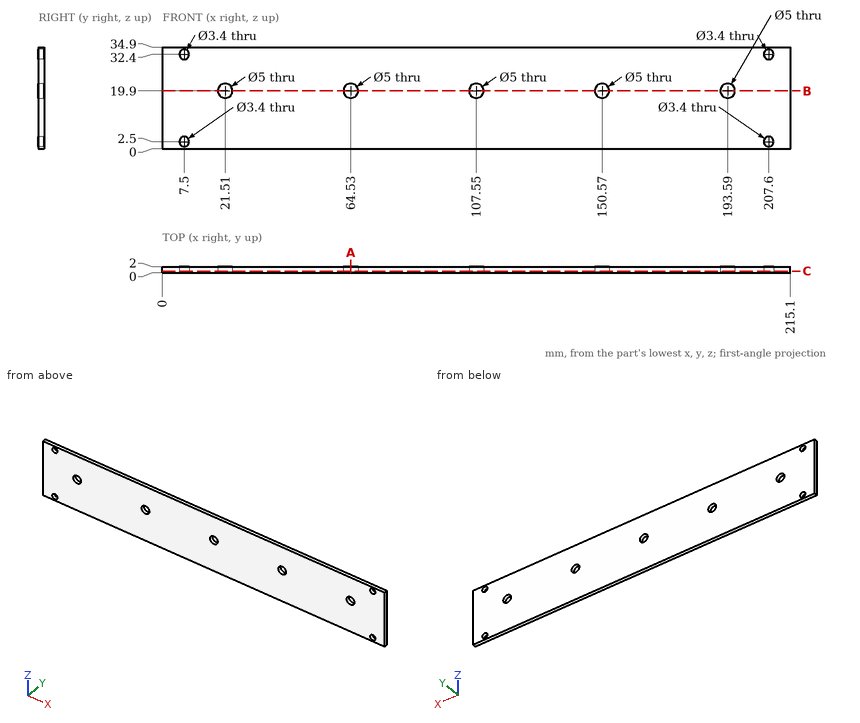
Source: three-view drawing plus pictorial views. Frame: mm from the lowest corner of the part. Round coordinates to 2 decimals unless told otherwise and drop trailing zeros. Write each loop counter-clockwise with the first axis right and the second up, starting at its lowest first coordinate (ties: lowest second). Pieces come first, ordered by that corner, then holes. Notation, with made-up numbers: (38, -26.5) -> (54, -26.5) arc R16 ccw to (54, -12.5) -> close; hole circle Ø10 at (-22, 29). An arc over 180 degrees is marked (long way). Return JSON: item names as keys, results as strings.
Q1. Section A-A on x = 64.53. Return the cut outline in (y, z), and give its area (3 significant figures).
From the geometry:
{"outline": "(0, 0) -> (2, 0) -> (2, 17.4) -> (0, 17.4) -> close; (0, 22.4) -> (2, 22.4) -> (2, 34.9) -> (0, 34.9) -> close", "area": "59.8 mm2"}
Q2. Ray query, line 1 (X direction, y = 1.1, z = 19.9); line 2 (X direction, y = 1.5, z = 32.4); line 3 (Z direction, x = 7.5, y = 1.55). Return the intervals inside material, ascending.
From the geometry:
{"line 1": "0 to 19.01, 24.01 to 62.03, 67.03 to 105.05, 110.05 to 148.07, 153.07 to 191.09, 196.09 to 215.1", "line 2": "0 to 5.8, 9.2 to 205.9, 209.3 to 215.1", "line 3": "0 to 0.8, 4.2 to 30.7, 34.1 to 34.9"}
Q3. Section C-C on y = 0.6. Give the number of separate pieces and of enclosed holes in the cut face, and give its area (3 significant figures).
From the geometry:
{"separate pieces": "1", "enclosed holes": "9", "area": "7,370 mm2"}
Q4. First-contact query: pin 1 Ø4.5 at (x, z) = (107.55, 19.9) entering from +Y; pin 2 Ø6 at (x, z) = (64.53, 19.9) entering from -Y. Flat tips, straight axial feed; report the tip coordinate or a pass-through.
From the geometry:
{"pin 1": "through", "pin 2": "y = 0"}
Q5. Section B-B on z = 19.9. Return the cut outline in (x, y), and give its area (3 significant figures).
From the geometry:
{"outline": "(0, 0) -> (19.01, 0) -> (19.01, 2) -> (0, 2) -> close; (24.01, 0) -> (62.03, 0) -> (62.03, 2) -> (24.01, 2) -> close; (67.03, 0) -> (105.05, 0) -> (105.05, 2) -> (67.03, 2) -> close; (110.05, 0) -> (148.07, 0) -> (148.07, 2) -> (110.05, 2) -> close; (153.07, 0) -> (191.09, 0) -> (191.09, 2) -> (153.07, 2) -> close; (196.09, 0) -> (215.1, 0) -> (215.1, 2) -> (196.09, 2) -> close", "area": "380 mm2"}
